Input: part model. Units: mm. Frame: model coordinates. A direction names the side the tool comes from. Round coordinates to 2 decimals unless told otherwise and drop trailing zeros. Loops run counter-clockwise (first coordinate to the right, second up) from the corner with the lowest first, then second, coordinate; pieces in that order, holes last. Notation, with made-up numbers: M 16,-32 L 42,-32 A12 ccw 42,-11 Z; hole C -12,28 d2. An arc over 180 degrees is marked long. Return JSON: item names as keys, results as strings. Group by question number.
1) Material intervals for line 1 (Y direction, x = -37.5, z = -2.5); line 2 (Y direction, x = -33.5, z = 1.25); line 3 (Y direction, x = -12, z = 2.25), sorted ascending. Write a range as from..to.
2) Access query for faces 1 (the face through (-37.79, 4.54, -1.97)), 2 (the face through (-1, 30.723, 1)), 3 (the face through (-1, -8, 3)). Directions: +Z, -Z, +X, -X, +Y, -Y. A direction counts if a zero-diameter tool reaches every point of the face in a straight line with its end or side. Return the directions, or none.
3) Section B-B (z = -1). Output: boundary loops of the cut face in (x, y).
4) Section D-D (x = -37.5). Output: boundary loops of the cut face in (y, z).
5) Mould query, pull axis X, two halves, no side actions, for faces 4 (the face through (34.503, 34.091, -1.972)), 5 (the face through (-40.497, 34.091, -1.972)), 6 (the face through (48.25, -1, 1)), 7 (the face through (-1, -38.25, 1)). Classes: +X half, -X half, draft (parallel to the pull), parting line (faces both ways), or undercut.
6) Section C-C (y = 16.5). Output: boundary loops of the cut face in (x, z).
7) Contact query for a flat-ended pin moving along its axis: P1, Ø0.8, axis at x = 38, y = 34.5, coming from the -Z side. Output: stop coordinate, or through.
8) Section A-A (x = 12.5). Output: boundary loops of the cut face in (y, z).
from build123d import *

# Parameters (mm, degrees)
SKETCH_W      = 96.5
SKETCH_H      = 76.5
SKETCH_R      = 1.75
SKETCH_R_2    = 2.2
SKETCH_R_3    = 3.370836
SKETCH_W_2    = 71.5
SKETCH_H_2    = 24.5
PAD_DEPTH     = 3
SKETCH001_R   = 3
SKETCH001_R_2 = 1.35
PAD001_DEPTH  = 4


with BuildPart() as part:
    # Sketch → Pad (new body)
    with BuildSketch(Plane.XY):
        Rectangle(SKETCH_W, SKETCH_H)
        with Locations((-43, -10.25)):
            Circle(SKETCH_R, mode=Mode.SUBTRACT)
        with Locations((43, -10.25)):
            Circle(SKETCH_R, mode=Mode.SUBTRACT)
        with Locations((-30.747, -7.700343)):
            Circle(SKETCH_R_2, mode=Mode.SUBTRACT)
        with Locations((-10.747, -7.700343)):
            Circle(SKETCH_R_2, mode=Mode.SUBTRACT)
        with Locations((-30.747, -27.700343)):
            Circle(SKETCH_R_2, mode=Mode.SUBTRACT)
        with Locations((-10.747, -27.700343)):
            Circle(SKETCH_R_2, mode=Mode.SUBTRACT)
        with Locations((20.747, -17.700343)):
            Circle(SKETCH_R_3, mode=Mode.SUBTRACT)
        with Locations((0, 18.472892)):
            Rectangle(SKETCH_W_2, SKETCH_H_2, mode=Mode.SUBTRACT)
    extrude(amount=PAD_DEPTH)

    # Sketch001 (on Face16 of Pad) → Pad001 (join)
    with BuildSketch(Plane(origin=(0, 0, 0), x_dir=(1, 0, 0), z_dir=(0, 0, -1))):
        with Locations((-37.5, -3.222892)):
            Circle(SKETCH001_R)
        with Locations((-37.5, -3.222892)):
            Circle(SKETCH001_R_2, mode=Mode.SUBTRACT)
        with Locations((37.5, -3.222892)):
            Circle(SKETCH001_R)
        with Locations((37.5, -3.222892)):
            Circle(SKETCH001_R_2, mode=Mode.SUBTRACT)
        with Locations((37.5, -34.222892)):
            Circle(SKETCH001_R)
        with Locations((37.5, -34.222892)):
            Circle(SKETCH001_R_2, mode=Mode.SUBTRACT)
        with Locations((-37.5, -34.222892)):
            Circle(SKETCH001_R)
        with Locations((-37.5, -34.222892)):
            Circle(SKETCH001_R_2, mode=Mode.SUBTRACT)
    extrude(amount=PAD001_DEPTH)


solid = part.part
Returned:
{
 "1": {"line 1": "y = 0.22..1.87, 4.57..6.22, 31.22..32.87, 35.57..37.22", "line 2": "y = -38.25..6.22, 30.72..38.25", "line 3": "y = -38.25..-29.51, -25.89..-9.51, -5.89..6.22, 30.72..38.25"},
 "2": {"face 1": "-Z", "face 2": "+Z, -Z", "face 3": "+Z, +X, -X, +Y, -Y"},
 "3": {"outline": "C -37.5,3.22 d6; C -37.5,34.22 d6; C 37.5,3.22 d6; C 37.5,34.22 d6; hole C -37.5,3.22 d2.7; hole C -37.5,34.22 d2.7; hole C 37.5,3.22 d2.7; hole C 37.5,34.22 d2.7"},
 "4": {"outline": "M -38.25,0 L 0.22,0 L 0.22,-4 L 1.87,-4 L 1.87,0 L 4.57,0 L 4.57,-4 L 6.22,-4 L 6.22,0 L 31.22,0 L 31.22,-4 L 32.87,-4 L 32.87,0 L 35.57,0 L 35.57,-4 L 37.22,-4 L 37.22,0 L 38.25,0 L 38.25,3 L -38.25,3 Z"},
 "5": {"face 4": "undercut", "face 5": "undercut", "face 6": "+X half", "face 7": "draft"},
 "6": {"outline": "M -48.25,0 L -35.75,0 L -35.75,3 L -48.25,3 Z; M 35.75,0 L 48.25,0 L 48.25,3 L 35.75,3 Z"},
 "7": {"P1": "stops at z = 0"},
 "8": {"outline": "M -38.25,0 L 6.22,0 L 6.22,3 L -38.25,3 Z; M 30.72,0 L 38.25,0 L 38.25,3 L 30.72,3 Z"}
}
